from build123d import *

# Parameters (mm, degrees)
F0_W     = 304.8
F0_H     = 355.6
F0_W_2   = 33.02
F0_H_2   = 33.02
F1_DEPTH = 25.4
F3_DEPTH = 25.401
F4_R     = 5.08
F5_W     = 104.775
F5_H     = 104.775
F6_DEPTH = 6.35
F7_R     = 5.08


with BuildPart() as f1:
    # F0 (on Top) → F1 (new body)
    with BuildSketch(Plane.XY):
        Rectangle(F0_W, F0_H)
        Rectangle(F0_W_2, F0_H_2, mode=Mode.SUBTRACT)
    extrude(amount=F1_DEPTH)

    # F2 (on face) → F3 (cut, through all)
    with BuildSketch(Plane.XY.offset(25.4)):
        with BuildLine():
            Line((69.737374, -127), (-82.430303, -127))
            ThreePointArc((-82.430303, -127), (-101.480303, -146.05), (-82.430303, -165.1))
            Line((-82.430303, -165.1), (69.737374, -165.1))
            ThreePointArc((69.737374, -165.1), (89.021114, -146.05), (69.737374, -127))
        make_face()
    extrude(amount=-F3_DEPTH, mode=Mode.SUBTRACT)

    # F4
    f4_edges = [f1.edges().sort_by_distance(p)[0] for p in [
        (0, -177.8, 25.4),
        (0, -177.8, 0),
        (152.4, 0, 25.4),
        (152.4, 0, 0),
        (-152.4, 0, 25.4),
        (-152.4, 0, 0),
        (0, 177.8, 0),
        (-6.346464, -127, 25.4),
        (-101.480303, -146.05, 25.4),
        (89.021114, -146.05, 25.4),
        (-6.346464, -165.1, 0),
        (89.021114, -146.05, 0),
        (0, 177.8, 25.4),
        (152.4, 177.8, 12.7),
        (-152.4, 177.8, 12.7),
        (-152.4, -177.8, 12.7),
        (152.4, -177.8, 12.7),
    ]]
    fillet(f4_edges, radius=F4_R)

    # F5 (on face) → F6 (cut)
    with BuildSketch(Plane(origin=(0, 0, 0), x_dir=(1, 0, 0), z_dir=(0, 0, -1))):
        Rectangle(F5_W, F5_H)
    extrude(amount=-F6_DEPTH, mode=Mode.SUBTRACT)

    # F7
    f7_edges = [f1.edges().sort_by_distance(p)[0] for p in [
        (-52.3875, -52.3875, 3.175),
        (52.3875, -52.3875, 3.175),
        (-52.3875, 52.3875, 3.175),
        (52.3875, 52.3875, 3.175),
    ]]
    fillet(f7_edges, radius=F7_R)


solid = f1.part
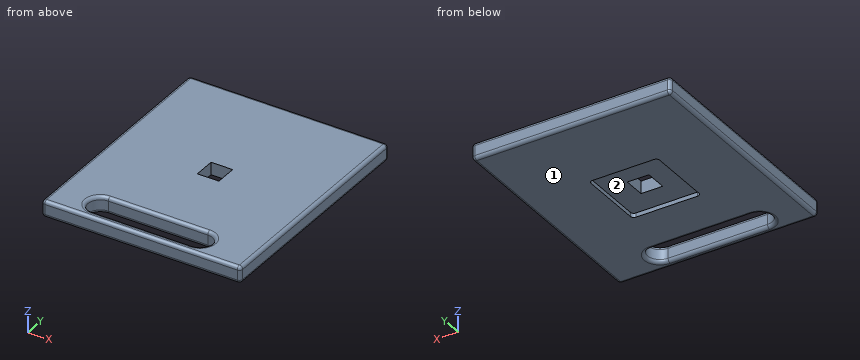
Can you work these out from the model? Positions are in its coordinate system, mm. Face numbers are marked on the shaded views. Coordinates: 2 decimals unless noted, no trailing zeros. Order: outer loops, then holes, each group sorted by start corner. A loop starts at its lowest first (then second) coordinate and runs counter-clockwise, first axis right, second up. Notation, with made-up numbers: M -20,10 L 37,10 A26 cw 37,38 Z; hole C 20,49 d8. An arc over 180 degrees is marked long. Write item = value, one per line.
(1) I need wall thicknesses on line 1 along Y through (x, z) = (20, 19.75); line 2 along X through (y, z) = (-41, 5.75); line 3 along X through (y, z) = (-142, 3.25). Which ranges of each line are inside material? Lowest first, please. Write a range as [from, to].
Results are:
line_1 = [-177.8, -165.1], [-127, 177.8]
line_2 = [-152.4, -52.39], [52.39, 152.4]
line_3 = [-152.06, -101.39], [88.93, 152.06]
(2) If we mould it in two halves opening along X, with no side actions, what happens to the marked faces 1 and 2? For each: pulls with the +X half, pulls with the -X half, needs draft (parallel to the pull), parting line crosses it, or undercut.
Results are:
face_1 = needs draft
face_2 = undercut
(3) Suppose I cut it at A-A on x = -78. Please give me the cut outline in (y, z).
Results are:
outline = M -177.8,5.08 A5.08 ccw -172.72,0 L -170.18,0 A5.08 ccw -165.1,5.08 L -165.1,20.32 A5.08 ccw -170.18,25.4 L -172.72,25.4 A5.08 ccw -177.8,20.32 Z; M -127,5.08 A5.08 ccw -121.92,0 L 172.72,0 A5.08 ccw 177.8,5.08 L 177.8,20.32 A5.08 ccw 172.72,25.4 L -121.92,25.4 A5.08 ccw -127,20.32 Z
(4) Suppose I cut it at B-B on x = 2. Please give me the cut outline in (y, z).
Results are:
outline = M -177.8,5.08 A5.08 ccw -172.72,0 L -170.18,0 A5.08 ccw -165.1,5.08 L -165.1,20.32 A5.08 ccw -170.18,25.4 L -172.72,25.4 A5.08 ccw -177.8,20.32 Z; M -127,5.08 A5.08 ccw -121.92,0 L -52.39,0 L -52.39,6.35 L -16.51,6.35 L -16.51,25.4 L -121.92,25.4 A5.08 ccw -127,20.32 Z; M 16.51,6.35 L 52.39,6.35 L 52.39,0 L 172.72,0 A5.08 ccw 177.8,5.08 L 177.8,20.32 A5.08 ccw 172.72,25.4 L 16.51,25.4 Z
(5) For pin 1 Ø3 at (y, z) = (-4.5, 2.5) entering from -X, with a flat end and sliding along its axis, tell me the tip position at first contact or that it passes through.
Results are:
pin_1 = -152.28
(6) Suppose I cut it at C-C on z = 12.5. Please give me the cut outline in (x, y), plus the area to 3 significant figures.
Results are:
outline = M -152.4,-172.72 A5.08 ccw -147.32,-177.8 L 147.32,-177.8 A5.08 ccw 152.4,-172.72 L 152.4,172.72 A5.08 ccw 147.32,177.8 L -147.32,177.8 A5.08 ccw -152.4,172.72 Z; hole M -82.43,-165.1 L 69.74,-165.1 A19.05 ccw long 69.74,-127 L -82.43,-127 A19.05 ccw Z; hole M -16.51,-16.51 L 16.51,-16.51 L 16.51,16.51 L -16.51,16.51 Z
area = 100,000 mm2
